from build123d import *

# Parameters (mm, degrees)
SKETCH_1_R          = 2
EXTRUDE_1_DEPTH     = 2
SKETCH_2_R          = 1
SKETCH_2_R_2        = 1.7
SKETCH_2_R_3        = 35
SKETCH_2_R_4        = 3
SKETCH_2_W          = 7
SKETCH_2_H          = 24
CUT_EXTRUDE_1_DEPTH = 10


with BuildPart() as part:
    # 草图1 → 凸台-拉伸1 (new body)
    with BuildSketch(Plane(origin=(0, 0, 0), x_dir=(1, 0, 0), z_dir=(0, 1, 0))):
        Polygon((0, -9.790421162), (0, 144.54053128), (31.526911935, 176.067443214), (185.857864376, 176.067443214), (217.384776311, 144.54053128), (217.384776311, -9.790421162), (185.857864376, -41.317333096), (31.526911935, -41.317333096), align=None)
        with Locations((68.692388155, 163.08216184)):
            Circle(SKETCH_1_R, mode=Mode.SUBTRACT)
        with Locations((148.692388155, 163.08216184)):
            Circle(SKETCH_1_R, mode=Mode.SUBTRACT)
        with Locations((204.399494937, 107.375055059)):
            Circle(SKETCH_1_R, mode=Mode.SUBTRACT)
        with Locations((204.399494937, 27.375055059)):
            Circle(SKETCH_1_R, mode=Mode.SUBTRACT)
        with Locations((148.692388155, -28.332051722)):
            Circle(SKETCH_1_R, mode=Mode.SUBTRACT)
        with Locations((68.692388155, -28.332051722)):
            Circle(SKETCH_1_R, mode=Mode.SUBTRACT)
        with Locations((12.985281374, 27.375055059)):
            Circle(SKETCH_1_R, mode=Mode.SUBTRACT)
        with Locations((12.985281374, 107.375055059)):
            Circle(SKETCH_1_R, mode=Mode.SUBTRACT)
    extrude(amount=EXTRUDE_1_DEPTH)

    # 草图2 → 切除-拉伸1 (cut)
    with BuildSketch(Plane(origin=(0, 2, 0), x_dir=(1, 0, 0), z_dir=(0, 1, 0))):
        with Locations((9.25, 96.625055059)):
            Circle(SKETCH_2_R)
        with Locations((108.692388155, 116.625055059)):
            Circle(SKETCH_2_R_2)
        with Locations((108.692388155, 18.125055059)):
            Circle(SKETCH_2_R_2)
        with Locations((157.942388155, 67.375055059)):
            Circle(SKETCH_2_R_2)
        with Locations((59.442388155, 67.375055059)):
            Circle(SKETCH_2_R_2)
        with Locations((108.692388155, 67.375055059)):
            Circle(SKETCH_2_R_3)
        with Locations((32.75, 96.625055059)):
            Circle(SKETCH_2_R)
        with Locations((32.75, 71.125055059)):
            Circle(SKETCH_2_R)
        with Locations((9.25, 71.125055059)):
            Circle(SKETCH_2_R)
        with Locations((25.58, 63.125055059)):
            Circle(SKETCH_2_R)
        with Locations((25.58, 37.625055059)):
            Circle(SKETCH_2_R)
        with Locations((108.692388155, -6.317333096)):
            Circle(SKETCH_2_R_4)
        Polygon((29, 97.375055059), (34, 92.375055059), (34, 75.375055059), (29, 70.375055059), (13, 70.375055059), (8, 75.375055059), (8, 92.375055059), (13, 97.375055059), align=None)
        with Locations((20.5, 50.375055059)):
            Rectangle(SKETCH_2_W, SKETCH_2_H)
        with BuildLine():
            Line((173.213203436, 23.682666904), (181.556349186, 23.682666904))
            ThreePointArc((181.556349186, 23.682666904), (182.321716051, 23.834907839), (182.970562748, 24.268453341))
            Line((182.970562748, 24.268453341), (186.798989873, 28.096880466))
            ThreePointArc((186.798989873, 28.096880466), (187.232535376, 28.745727164), (187.384776311, 29.511094028))
            Line((187.384776311, 29.511094028), (187.384776311, 47.854239779))
            ThreePointArc((187.384776311, 47.854239779), (187.232535376, 48.619606644), (186.798989873, 49.268453341))
            Line((186.798989873, 49.268453341), (182.970562748, 53.096880466))
            ThreePointArc((182.970562748, 53.096880466), (182.321716051, 53.530425969), (181.556349186, 53.682666904))
            Line((181.556349186, 53.682666904), (173.213203436, 53.682666904))
            ThreePointArc((173.213203436, 53.682666904), (172.447836571, 53.530425969), (171.798989873, 53.096880466))
            Line((171.798989873, 53.096880466), (167.970562748, 49.268453341))
            ThreePointArc((167.970562748, 49.268453341), (167.537017246, 48.619606644), (167.384776311, 47.854239779))
            Line((167.384776311, 47.854239779), (167.384776311, 29.511094028))
            ThreePointArc((167.384776311, 29.511094028), (167.537017246, 28.745727164), (167.970562748, 28.096880466))
            Line((167.970562748, 28.096880466), (171.798989873, 24.268453341))
            ThreePointArc((171.798989873, 24.268453341), (172.447836571, 23.834907839), (173.213203436, 23.682666904))
        make_face()
    extrude(amount=-CUT_EXTRUDE_1_DEPTH, mode=Mode.SUBTRACT)


solid = part.part
Geometry check sheet. Reference: the model listing, model coordinates, mm. A direction names the side the tool comes from. Give positions to 0.01 mm unless a question says otherwise; leave off trailing zeros. Loops run counter-clockwise (first coordinate to the right, second up) from the corner with the lowest first, then second, coordinate; pieces in that order, holes last. Notation, with made-up numbers: M -20.75,74.25 L 27.25,74.25 A23 cw 27.25,87.25 Z; hole C 36,-30.5 d11. An arc over 180 degrees is marked long. Write each question's results on one line, items separated by ' | '.
1) Section check B-B, the plane z = -152. Record the boundary of the cut face in (x, y), plus the area to 3 significant figures.
Answers follow:
outline: M 7.46,0 L 209.93,0 L 209.93,2 L 7.46,2 Z | area: 405 mm2
2) Section check C-C, the plane y = 0.3. Count the separate pieces of the cut face and the enclosed holes in it, plus the area to 3 significant figures.
Answers follow:
separate pieces: 1 | enclosed holes: 23 | area: 39,900 mm2
3) Release check for a two-part mould opening along X. For faces 1 (the face through (15.54, 0.99, -160.08)), 2 (the face through (31.535, 1.014, -72.91)), 3 (the face through (201.401, 0.986, -160.525)) record: +X half, -X half, draft (parallel to the pull), parting line (faces both ways), or undercut.
Answers follow:
face 1: -X half | face 2: undercut | face 3: +X half
4) Thickness scan on line 1 (X direction, y = 1.75, z = -92.5); line 2 (Z direction, x = 11.5, y = 1.4); line 3 (X direction, y = 0.5, z = -116.5). Record the ranges inside material, lowest first.
Answers follow:
line 1: 0 to 8.12, 33.88 to 84.33, 133.06 to 217.38 | line 2: -156.04 to -108.71, -106.04 to -95.88, -71.88 to -28.71, -26.04 to 21.29 | line 3: 0 to 107, 110.39 to 217.38
5) Gauge pin test, flat ends, axial feed: pin 1 (2 mm diameter, centred on x = 145.5, z = -28.5, fed in from -Y); pin 2 (0.6 mm diameter, centred on x = 20.5, y = 0.5, fed in from +Z). Record the tip position at first contact, or that the pin passes through.
Answers follow:
pin 1: y = 0 | pin 2: z = 30.59
6) Section check A-A, the plane x = 98.5. Record the boundary of the cut face in (y, z).
Answers follow:
outline: M 0,-176.07 L 2,-176.07 L 2,-100.86 L 0,-100.86 Z; M 0,-33.89 L 2,-33.89 L 2,41.32 L 0,41.32 Z
7) Tool access check on faces 4 (the face through (134, 0, -93)), 5 (the face through (31.465, 1.014, -94.91)). Record the directions out of +Z, -Z, +X, -X, +Y, -Y that give a thin tool (end or side, any length) a straight path to the whole face; none if there is none.
Answers follow:
face 4: +Z, -Z, +X, -X, -Y | face 5: +Y, -Y
